Geometry: see drawing. Coordinates: mm, zero at the bounding-box minimum. A direction names the side the tool comes from. Coordinates: 2 decimals unless noted, no trailing zeros. Order: outer loops, then holes, each group sorted by start corner. A loop starts at its lowest first (then second) coordinate and runs counter-clockwise, first axis right, second up.
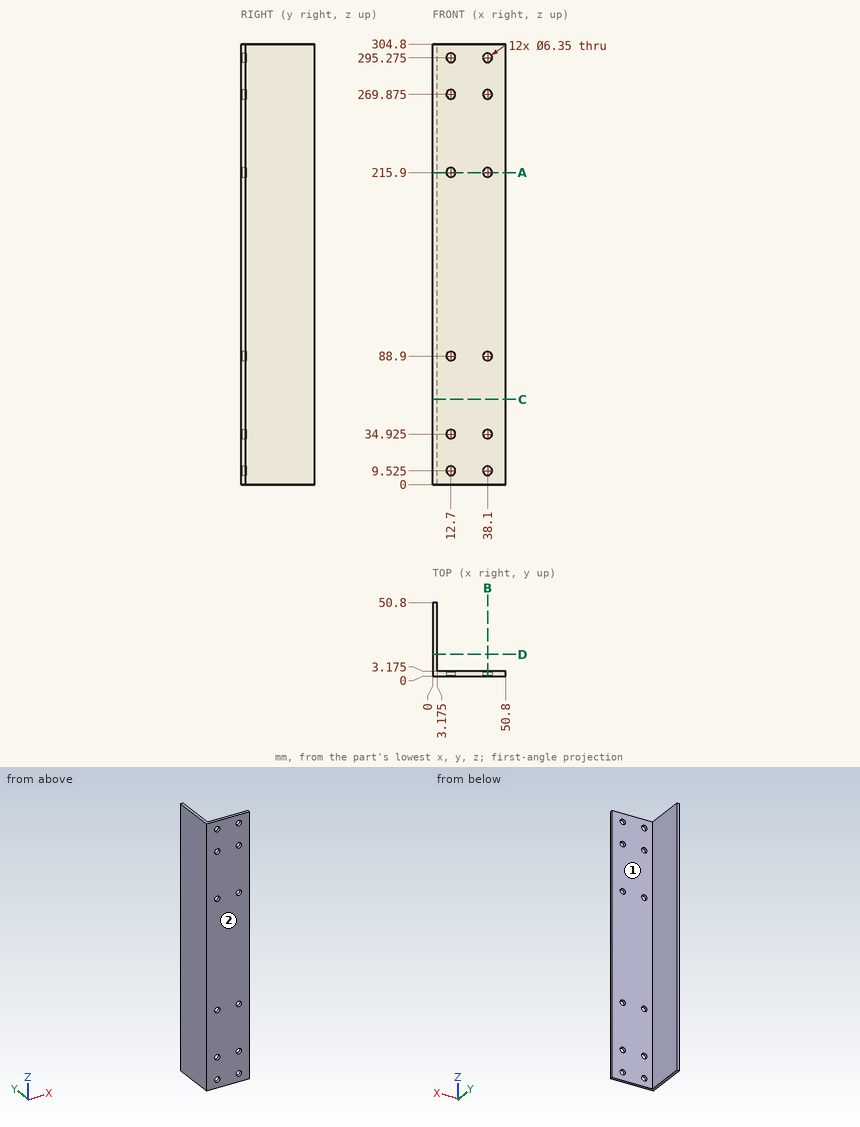
Q1. Material intervals for line 1 along X through (y, z) = (1.8, 88.9) (3 decimals); line 2 along Y through (x, z) = (31.5, 144) (3 decimals), sorted ascending.
Solutions:
line 1: x = 0 to 9.525, 15.875 to 34.925, 41.275 to 50.8
line 2: y = 0 to 3.175
Q2. Set-up query: the marked faces 1 and 2. Return all of +Z, -Z, +X, -X, +Y, -Y with unobstructed straight access to the full face (end or side cutting, diameter ignored); none if empty.
Solutions:
face 1: +Z, -Z, +X, +Y
face 2: +Z, -Z, +X, -X, -Y
Q3. Pin query (flat end, axial travel): P1, Ø10, axis at y = 40.5, z = 171.5, coming from the +X side (3 decimals); P2, Ø8.5, axis at x = 38.1, z = 88.9, coming from the +Y side (3 decimals). Return the tip coordinate at first contact, or that it passes through.
Solutions:
P1: stops at x = 3.175
P2: stops at y = 3.175
Q4. Section query D-D on y = 15. Output: boundary loops of the cut face in (x, z) (3 decimals), plus the area to 3 significant figures.
Solutions:
outline: (0, 0) - (3.175, 0) - (3.175, 304.8) - (0, 304.8) - close
area: 968 mm2
Q5. Section query A-A on z = 215.9. Output: boundary loops of the cut face in (x, y) (3 decimals).
Solutions:
outline: (0, 0) - (9.525, 0) - (9.525, 3.175) - (3.175, 3.175) - (3.175, 50.8) - (0, 50.8) - close; (15.875, 0) - (34.925, 0) - (34.925, 3.175) - (15.875, 3.175) - close; (41.275, 0) - (50.8, 0) - (50.8, 3.175) - (41.275, 3.175) - close
Q6. Section query B-B on x = 38.1. Output: boundary loops of the cut face in (y, z) (3 decimals), plus the area to 3 significant figures.
Solutions:
outline: (0, 0) - (3.175, 0) - (3.175, 6.35) - (0, 6.35) - close; (0, 12.7) - (3.175, 12.7) - (3.175, 31.75) - (0, 31.75) - close; (0, 38.1) - (3.175, 38.1) - (3.175, 85.725) - (0, 85.725) - close; (0, 92.075) - (3.175, 92.075) - (3.175, 212.725) - (0, 212.725) - close; (0, 219.075) - (3.175, 219.075) - (3.175, 266.7) - (0, 266.7) - close; (0, 273.05) - (3.175, 273.05) - (3.175, 292.1) - (0, 292.1) - close; (0, 298.45) - (3.175, 298.45) - (3.175, 304.8) - (0, 304.8) - close
area: 847 mm2
Q7. Section query C-C on z = 59. Output: boundary loops of the cut face in (x, y) (3 decimals).
Solutions:
outline: (0, 0) - (50.8, 0) - (50.8, 3.175) - (3.175, 3.175) - (3.175, 50.8) - (0, 50.8) - close
